The figure shows three views and two pictorial views of one solid part (mm, origin at its lowest corner). Answer the questions. Give positions to 0.01 mm unless a question says otherwise; leave off trailing zeros. Loops run counter-clockwise (first coordinate to the right, second up) from the corner with the lowest first, then second, coordinate; pieces in that order, holes last. Notation, with made-up numbers: (37.25, 76.5) - (74.25, 76.5) arc R23 ccw to (74.25, 107.5) - close; hole circle Ø10 at (-20.75, 54.25). An arc over 180 degrees is marked (long way). Use a Markdown table: item, result. Add a question column.
Item 1: A cutting plane is placed at D-D (x = 74.5). Determine the outline of the cut face in (y, z), plus the area to 3 significant figures.
Item 2: A cutting plane is placed at A-A (z = 1.75). Determine the outline of the cut face in (x, y), plus the area to 3 significant figures.
Item 3: A cutting plane is placed at B-B (x = 40). Determine the outline of the cut face in (y, z), plus the area to 3 significant figures.
Item 4: Consider probe 1 along X at (y, z) = (7, 2.55); probe 2 along X at (y, z) = (6.5, 1.7); probe 3 along Y at (x, z) = (41.5, 1.3). Determine where each line is inside the solid, lowest interval first. Write a range as [from, to].
Item 5: Each of these flat-tipped pins is pushed along its axis until it touches: P1, Ø1, axis at y = 42.5, z = 1, coming from the -X side; P2, Ø0.9, axis at y = 6.5, z = 1.5, coming from the -X side; P3, Ø1.5, axis at y = 63, z = 1, coming from the -X side. Where does it stop, or does it pass through?
Item 6: A cutting plane is placed at C-C (y = 66). Determine the outline of the cut face in (x, z).
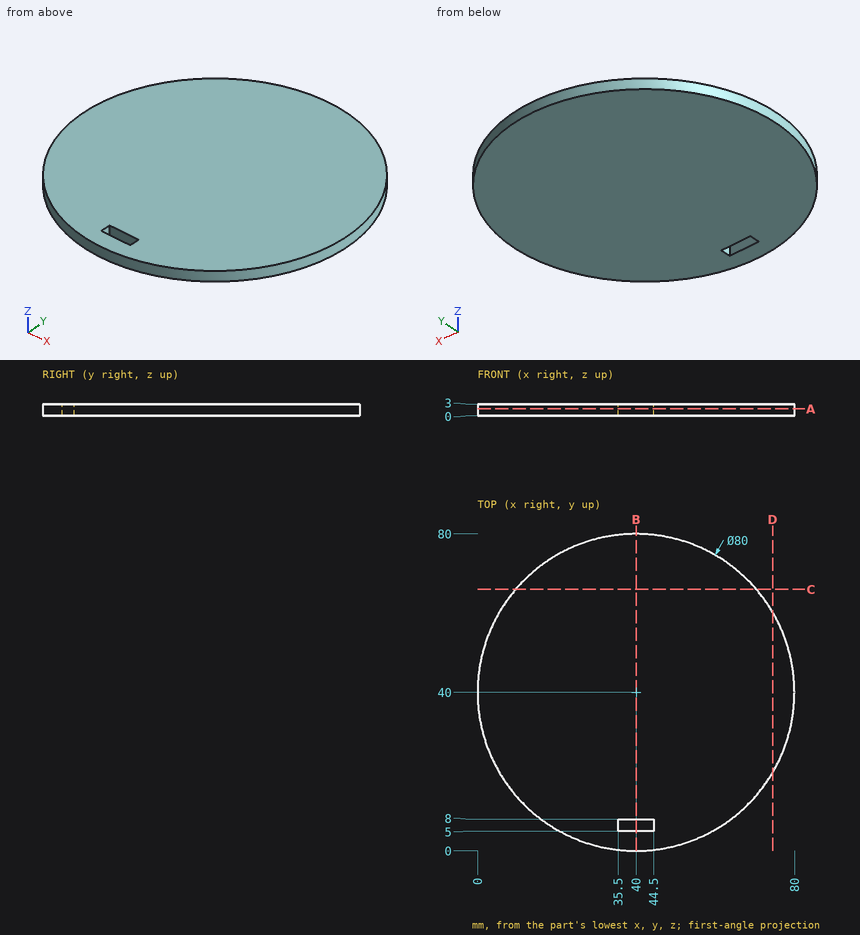
Geometry says:
| question | item | result |
|---|---|---|
| 1 | outline | (19.76, 0) - (60.24, 0) - (60.24, 3) - (19.76, 3) - close |
| 1 | area | 121 mm² |
| 2 | outline | circle Ø80 at (40, 40); hole (35.5, 5) - (44.5, 5) - (44.5, 8) - (35.5, 8) - close |
| 2 | area | 5,000 mm² |
| 3 | outline | (0, 0) - (5, 0) - (5, 3) - (0, 3) - close; (8, 0) - (80, 0) - (80, 3) - (8, 3) - close |
| 3 | area | 231 mm² |
| 4 | probe 1 | [17.39, 35.5], [44.5, 62.61] |
| 4 | probe 2 | [18.14, 35.5], [44.5, 61.86] |
| 4 | probe 3 | [0.03, 5], [8, 79.97] |
| 5 | P1 | x = 0.05 |
| 5 | P2 | x = 17.47 |
| 5 | P3 | x = 6.76 |
| 6 | outline | (9.6, 0) - (70.4, 0) - (70.4, 3) - (9.6, 3) - close |
